Build history of the part. All positions in model axes, mm. A direction names the side the tool comes from. Round coordinates to 2 decimals unless told otherwise and drop trailing zeros. Write each loop counter-clockwise with the first axis right and the second up, starting at its lowest first coordinate (ties: lowest second). Pieces come first, ordered by that corner, then holes. Notation, with made-up numbers: (20.5, 33.5) -> (75.5, 33.5) arc R8 cw to (75.5, 38.5) -> close; hole circle Ø1 at (26, 83.25). An arc over 180 degrees is marked (long way). Return JSON: item names as keys, results as strings.
from build123d import *

# Parameters (mm, degrees)
BOSS_EXTRU_1_DEPTH      = 191
ENL_V_MAT_EXTRU_1_DEPTH = 204.406327378
ESQUISSE2_R             = 53
ESQUISSE2_R_2           = 1
BOSS_EXTRU_2_DEPTH      = 5
BOSS_EXTRU_3_DEPTH      = 7
BOSS_EXTRU_4_DEPTH      = 7


with BuildPart() as part:
    # Esquisse1 → Boss.-Extru.1 (new body)
    with BuildSketch(Plane.XY):
        with BuildLine():
            Line((-17.5, -48.310889132), (-17.5, -47.310889132))
            ThreePointArc((-17.5, -47.310889132), (-9, -15.588457268), (-32.222431864, -38.810889132))
            Line((-32.222431864, -38.810889132), (-33.088457268, -39.310889132))
            ThreePointArc((-33.088457268, -39.310889132), (-35.314540075, -27.733649929), (-29.89862988, -17.26198201))
            ThreePointArc((-29.89862988, -17.26198201), (-41.675315415, -16.716463864), (-50.588457268, -9))
            Line((-50.588457268, -9), (-49.722431864, -8.5))
            ThreePointArc((-49.722431864, -8.5), (-18, 0), (-49.722431864, 8.5))
            Line((-49.722431864, 8.5), (-50.588457268, 9))
            ThreePointArc((-50.588457268, 9), (-44, 15.588457268), (-35, 18))
            Line((-35, 18), (35, 18))
            ThreePointArc((35, 18), (44, 15.588457268), (50.588457268, 9))
            Line((50.588457268, 9), (49.722431864, 8.5))
            ThreePointArc((49.722431864, 8.5), (18, 0), (49.722431864, -8.5))
            Line((49.722431864, -8.5), (50.588457268, -9))
            ThreePointArc((50.588457268, -9), (41.675315415, -16.716463864), (29.89862988, -17.26198201))
            ThreePointArc((29.89862988, -17.26198201), (35.314540075, -27.733649929), (33.088457268, -39.310889132))
            Line((33.088457268, -39.310889132), (32.222431864, -38.810889132))
            ThreePointArc((32.222431864, -38.810889132), (9, -15.588457268), (17.5, -47.310889132))
            Line((17.5, -47.310889132), (17.5, -48.310889132))
            ThreePointArc((17.5, -48.310889132), (6.36077534, -44.450113792), (0, -34.523964019))
            ThreePointArc((0, -34.523964019), (-6.36077534, -44.450113792), (-17.5, -48.310889132))
        make_face()
    extrude(amount=BOSS_EXTRU_1_DEPTH)

    # Esquisse4 → Enlèv. mat.-Extru.1 (cut, through all)
    with BuildSketch(Plane.XY.offset(191)):
        Polygon((11.259686126, -14.497651553), (18.185177603, -2.502348447), (49.722431864, -8.5), (50.588457268, -9), (33.088457268, -39.310889132), (32.222431864, -38.810889132), align=None)
        Polygon((-33.088457268, -39.310889132), (-32.222431864, -38.810889132), (-11.259686126, -14.497651553), (-18.185177603, -2.502348447), (-49.722431864, -8.5), (-50.588457268, -9), align=None)
    extrude(amount=-ENL_V_MAT_EXTRU_1_DEPTH, mode=Mode.SUBTRACT)

    # Esquisse2 → Boss.-Extru.2 (add)
    with BuildSketch(Plane.XY.offset(191)):
        Circle(ESQUISSE2_R)
        with Locations((-35, 0)):
            Circle(ESQUISSE2_R_2, mode=Mode.SUBTRACT)
        with Locations((-17.5, -30.310889132)):
            Circle(ESQUISSE2_R_2, mode=Mode.SUBTRACT)
        with Locations((17.5, -30.310889132)):
            Circle(ESQUISSE2_R_2, mode=Mode.SUBTRACT)
        with Locations((35, 0)):
            Circle(ESQUISSE2_R_2, mode=Mode.SUBTRACT)
        Polygon((41.674038106, 8.559773091), (35.611860279, 12.059773091), (36.611860279, 13.791823898), (42.674038106, 10.291823898), align=None, mode=Mode.SUBTRACT)
        Polygon((7.361860279, -36.870662223), (6.361860279, -38.602713031), (12.424038106, -42.102713031), (13.424038106, -40.370662223), align=None, mode=Mode.SUBTRACT)
        Polygon((-35.611860279, 12.059773091), (-36.611860279, 13.791823898), (-42.674038106, 10.291823898), (-41.674038106, 8.559773091), align=None, mode=Mode.SUBTRACT)
        Polygon((-7.361860279, -36.870662223), (-6.361860279, -38.602713031), (-12.424038106, -42.102713031), (-13.424038106, -40.370662223), align=None, mode=Mode.SUBTRACT)
    extrude(amount=BOSS_EXTRU_2_DEPTH)

    # Esquisse5 → Boss.-Extru.3 (add)
    with BuildSketch(Plane(origin=(21.486860279, -12.405444566, 0), x_dir=(0, 0, -1), z_dir=(0.8660254037844384, -0.5000000000000006, 0))):
        Polygon((-196, -28.25), (-190.4, -28.25), (-190.4, -26.25), (-188.4, -26.25), (-188.4, -28.25), (-188.4, -30.25), (-196, -30.25), align=None)
        Polygon((-190.4, 26.25), (-188.4, 26.25), (-188.4, 28.25), (-188.4, 30.25), (-196, 30.25), (-196, 28.25), (-190.4, 28.25), align=None)
    extrude(amount=BOSS_EXTRU_3_DEPTH)

    # Esquisse6 → Boss.-Extru.4 (add)
    with BuildSketch(Plane(origin=(-21.486860279, -12.405444566, 0), x_dir=(0, 0, 1), z_dir=(-0.8660254037844384, -0.5000000000000006, 0))):
        Polygon((196, -28.25), (190.4, -28.25), (190.4, -26.25), (188.4, -26.25), (188.4, -28.25), (188.4, -30.25), (196, -30.25), align=None)
        Polygon((190.4, 26.25), (188.4, 26.25), (188.4, 28.25), (188.4, 30.25), (196, 30.25), (196, 28.25), (190.4, 28.25), align=None)
    extrude(amount=BOSS_EXTRU_4_DEPTH)


solid = part.part
Q1. Two-plate mould, pull along Z, no slides. Class faces 4 (the flat face through (0, 18, 94)), 5 (the flat face through (-1, 1, 196)), 6 (the flat face through (-10, -39, 188.4)), 7 (the flat face through (11, -38, 190.4)): +Z half, -Z half, draft (parallel to the pull), parting line (faces both ways), or undercut.
Verdict:
{"face 4": "draft", "face 5": "+Z half", "face 6": "-Z half", "face 7": "undercut"}
Q2. Saw through at C-C on y = -19. List the corners of the cut face in (x, z), then the cut area to 3 significant figures.
Verdict:
{"outline": "(-49.48, 191) -> (-4.81, 191) -> (-4.81, 0) -> (4.81, 0) -> (4.81, 191) -> (49.48, 191) -> (49.48, 196) -> (-49.48, 196) -> close", "area": "2,330 mm²"}
Q3. Saw through at D-D on y = 36. List the corners of the cut face in (x, z), then the cut area to 3 significant figures.
Verdict:
{"outline": "(-38.9, 191) -> (38.9, 191) -> (38.9, 196) -> (-38.9, 196) -> close", "area": "389 mm²"}
Q4. 3-axis set-ups, long thin cutter, end or side, ignore diameter. For faces 1 (the flat face through (-39, 10, 188.4)), 2 (the flat face through (-14.674, -8.584, 96.837)), 3 (the flat face through (-38, 9, 190.4)): which of +Z, -Z, +X, -X, +Y, -Y reach the whole face in a straight line?
Verdict:
{"face 1": "-Z, -Y", "face 2": "-Z, -X", "face 3": "-Y"}
Q5. Saw through at B-B on x = -25. List the corners of the cut face in (y, z), then the cut area to 3 significant figures.
Verdict:
{"outline": "(-46.73, 191) -> (13.75, 191) -> (13.75, 0) -> (18, 0) -> (18, 191) -> (46.73, 191) -> (46.73, 196) -> (-46.73, 196) -> close", "area": "1,280 mm²"}
Q6. Wall check: L1, parallel to X at y = 9.5, z = 111; L2, parallel to Z at x = 35, y = -31; L3, parallel to Y at x = 21.5, z = 149.5. Give the ranges that are in metal, low to high.
Verdict:
{"L1": "x = -50.29 to -49.1, -20.9 to 20.9, 49.1 to 50.29", "L2": "z = 191 to 196", "L3": "y = 10.33 to 18"}
Q7. Saw through at A-A on z = 43.5. List the corners of the cut face in (x, y).
Verdict:
{"outline": "(-50.59, 9) -> (-49.72, 8.5) arc R17 cw to (-18.19, -2.5) -> (-11.26, -14.5) arc R17 cw to (-17.5, -47.31) -> (-17.5, -48.31) arc R18 ccw to (0, -34.52) arc R18 ccw to (17.5, -48.31) -> (17.5, -47.31) arc R17 cw to (11.26, -14.5) -> (18.19, -2.5) arc R17 cw to (49.72, 8.5) -> (50.59, 9) arc R18 ccw to (35, 18) -> (-35, 18) arc R18 ccw to start"}
Q8. Pin check, flat tips, straight feed: pin 1 Ø1.2 at (x, y) = (17.5, -30.31) entering from +Z; pin 2 Ø10 at (x, y) = (-32.5, 39) entering from -Z; pin 3 Ø8 at (x, z) = (-41.5, 102.5) entering from +Y; pin 4 Ø2 at (x, y) = (37.5, 12) entering from -Z. Stop position of each tip, or through.
Verdict:
{"pin 1": "passes through", "pin 2": "stops at z = 191", "pin 3": "stops at y = 17.83", "pin 4": "stops at z = 188.4"}
